Verification items for the finished model (mm, model axes). A direction names the side the tool comes from. Give positions to 0.01 mm unless a question says otherwise; leave off trailing zeros. Write each loop counter-clockwise with the first axis right and the second up, starting at its lowest first coordinate (ties: lowest second). Pieces come first, ordered by that corner, then holes. Notation, with made-up numbers: (-1, -18.75) - (20, -18.75) arc R15 cw to (20, 8.25) - close; hole circle Ø7 at (-35, 84). An arc over 180 degrees is marked (long way). Put each result on its own line as item: value.
Autodesk Inventor part; units mm, degrees
ref_plane "YZ Plane" through (0, 0, 0) normal (1, 0, 0) x (0, 1, 0)
ref_plane "XZ Plane" through (0, 0, 0) normal (0, 1, 0) x (-1, 0, 0)
ref_plane "XY Plane" through (0, 0, 0) normal (0, 0, 1) x (1, 0, 0)
sketch "Sketch1" plane through (0, 0, 0) normal (0, 0, 1) x (1, 0, 0)
  line L0 (-63.5, 0) -> (-368.3, 0)
  line L1 (-431.8, 63.5) -> (-431.8, 88.9)
  line L2 (-431.8, 88.9) -> (0, 88.9)
  line L3 (0, 88.9) -> (0, 63.5)
  arc A0 (-431.8, 63.5) -> (-368.3, 0) centre (-368.3, 63.5) ccw
  arc A1 (-63.5, 0) -> (0, 63.5) centre (-63.5, 63.5) ccw
  line L4 (-431.8, 88.9) -> (-287.8667, 88.9)
  line L5 (0, 88.9) -> (-143.9333, 88.9)
  point P0 (0, 0)
  point P1 (-431.8, 0)
  dimension "d0" = 431.8
  dimension "d1" = 88.9
  dimension "d2" = 63.5
  dimension "d3" = 63.5
extrude "Extrusion1" add sketch "Sketch1" along normal blind 23
sketch "Sketch2" plane through (0, 0, 23) normal (0, 0, 1) x (1, 0, 0)
  line L0 (-368.3, 0) -> (-63.5, 0)
  line L1 (0, 88.9) -> (-431.8, 88.9)
  line L2 (0, 63.5) -> (0, 88.9)
  line L3 (-431.8, 88.9) -> (-431.8, 63.5)
  point P0 (0, 0)
  point P1 (-368.3, 44.45)
  point P2 (-287.8667, 44.45)
  point P3 (-143.9333, 44.45)
  point P4 (-63.5, 44.45)
  dimension "d6" = 88.9
  dimension "d7" = 44.45
  dimension "d8" = 44.45
  dimension "d9" = 44.45
  dimension "d10" = 44.45
  dimension "d11" = 431.8
  dimension "d12" = 63.5
  dimension "d13" = 143.9333
  dimension "d14" = 143.9333
  dimension "d15" = 63.5
hole "Hole1" at (-368.3, 44.45, 23) at (-287.8667, 44.45, 23) at (-143.9333, 44.45, 23) at (-63.5, 44.45, 23) direction (0, 0, -1) diameter 7.9 end through all
sketch "Sketch3" plane through (-431.8, 88.9, 0) normal (0, 1, 0) x (1, 0, 0)
  line L0 (431.8, 0) -> (0, 0)
  line L1 (0, -23) -> (143.9333, -23)
  line L2 (143.9333, -23) -> (143.9333, 0)
  line L3 (143.9333, 0) -> (0, 0)
  line L4 (0, 0) -> (0, -23)
  line L5 (431.8, -23) -> (0, -23)
  line L6 (431.8, -23) -> (287.8667, -23)
  line L7 (287.8667, -23) -> (287.8667, 0)
  line L8 (287.8667, 0) -> (431.8, 0)
  line L9 (431.8, 0) -> (431.8, -23)
  dimension "d27" = 431.8
  dimension "d28" = 143.9333
  dimension "d29" = 143.9333
extrude "Extrusion2" add sketch "Sketch3" along normal blind 38.1 contours L9 L5 L7 L0 | L2 L1 L4 L0
sketch "Sketch4" plane through (0, 0, 23) normal (0, 0, 1) x (1, 0, 0)
  line L0 (-143.9333, 88.9) -> (-143.9333, 127)
  line L1 (-287.8667, 88.9) -> (-287.8667, 127)
  line L2 (-143.9333, 127) -> (0, 127)
  line L3 (-431.8, 127) -> (-287.8667, 127)
  circle A0 centre (-368.3, 44.45) radius 3.95
  circle A1 centre (-63.5, 44.45) radius 3.95
  point P0 (0, 0)
  point P1 (-63.5, 114.3)
  point P2 (-368.3, 114.3)
  dimension "d32" = 38.1
  dimension "d33" = 38.1
  dimension "d34" = 12.7
  dimension "d35" = 12.7
  dimension "d38" = 0
  dimension "d39" = 0
hole "Hole2" at (-63.5, 114.3, 23) at (-368.3, 114.3, 23) direction (0, 0, -1) diameter 11.9888 end through all
sketch "Sketch5" plane through (0, 0, 23) normal (0, 0, 1) x (1, 0, 0)
  circle A0 centre (-368.3, 114.3) radius 5.9944
  circle A1 centre (-63.5, 114.3) radius 5.9944
  point P0 (0, 0)
  point P1 (-360.553, 107.8738)
  point P2 (-375.3104, 98.806)
  point P3 (-388.7216, 106.553)
  point P4 (-71.247, 107.8738)
  point P5 (-56.4896, 98.806)
  point P6 (-43.0784, 106.553)
  dimension "d47" = 7.747
  dimension "d48" = 6.4262
  dimension "d49" = 7.0104
  dimension "d50" = 15.494
  dimension "d51" = 20.4216
  dimension "d52" = 7.747
  dimension "d53" = 7.747
  dimension "d54" = 6.4262
  dimension "d55" = 15.494
  dimension "d56" = 7.0104
  dimension "d57" = 7.747
  dimension "d58" = 20.4216
hole "Hole3" at (-360.553, 107.8738, 23) at (-375.3104, 98.806, 23) at (-388.7216, 106.553, 23) at (-71.247, 107.8738, 23) at (-56.4896, 98.806, 23) at (-43.0784, 106.553, 23) direction (0, 0, -1) diameter 3.175 end through all
equation "\"d28\" = 0.333333 * d27"
equation "\"d29\" = d28"
properties part number "side drivetrain piece (8 wheel macanum)"
Q1. Section check C-C, the plane y = 44.45. Record the cut outline in (x, z).
Answers follow:
outline: (-428.88, 0) - (-372.25, 0) - (-372.25, 23) - (-428.88, 23) - close; (-364.35, 0) - (-291.82, 0) - (-291.82, 23) - (-364.35, 23) - close; (-283.92, 0) - (-147.88, 0) - (-147.88, 23) - (-283.92, 23) - close; (-139.98, 0) - (-67.45, 0) - (-67.45, 23) - (-139.98, 23) - close; (-59.55, 0) - (-2.92, 0) - (-2.92, 23) - (-59.55, 23) - close
Q2. Section check A-A, the plane y = 114.3. Record the cut outline in (x, z), plus the area to 3 significant figures.
Answers follow:
outline: (-431.8, 0) - (-374.29, 0) - (-374.29, 23) - (-431.8, 23) - close; (-362.31, 0) - (-287.87, 0) - (-287.87, 23) - (-362.31, 23) - close; (-143.93, 0) - (-69.49, 0) - (-69.49, 23) - (-143.93, 23) - close; (-57.51, 0) - (0, 0) - (0, 23) - (-57.51, 23) - close
area: 6,070 mm2
Q3. Go/stop test with flat-tipped pins: pin 1 Ø5 at (y, z) = (46, 18) entering from -X; pin 2 Ø3.5 at (x, y) = (-56.49, 98.81) entering from -Z; pin 3 Ø10 at (y, z) = (38, 20.5) entering from +X; pin 4 Ø6 at (x, z) = (-248.5, 4.5) entering from +Y. Record where each tip stops, or that it passes through.
Answers follow:
pin 1: stops at x = -430
pin 2: stops at z = 0
pin 3: stops at x = -3.4
pin 4: stops at y = 88.9
Q4. Release check for a two-part mould opening along X. For faces 1 (the face through (-219, 64, 0)), 2 (the face through (0, 96, 11)), 3 (the face through (-287.867, 108, 12)) record: released by +X, released by -X, zero draft, split by the parting line, or undercut.
Answers follow:
face 1: zero draft
face 2: released by +X
face 3: undercut
Q5. Set-up check for faces 4 (the face through (-143.933, 108, 12)), 5 (the face through (-361, 127, 11)): record each of +Z, -Z, +X, -X, +Y, -Y from which the full face is reachable in a straight line by a thin tool's end or side.
Answers follow:
face 4: +Z, -Z, +Y
face 5: +Z, -Z, +X, -X, +Y
Q6. Section check D-D, the plane x = -184.5. Record the cut outline in (y, z).
Answers follow:
outline: (0, 0) - (88.9, 0) - (88.9, 23) - (0, 23) - close
Q7. Section check B-B, the plane z = 6.25. Give the number of separate pieces and of enclosed holes in the cut face, plus the area to 3 significant figures.
Answers follow:
separate pieces: 1
enclosed holes: 12
area: 47,200 mm2
Q8. Scan lines: line 1 along X through (y, z) = (115, 19.75); line 2 along Y through (x, z) = (-368.3, 5.5); line 3 along X through (y, z) = (117.5, 22). Record each from-to range of solid material in increasing order.
Answers follow:
line 1: x = -431.8 to -374.25, -362.35 to -287.87, -143.93 to -69.45, -57.55 to 0
line 2: y = 0 to 40.5, 48.4 to 108.31, 120.29 to 127
line 3: x = -431.8 to -373.37, -363.23 to -287.87, -143.93 to -68.57, -58.43 to 0
